from build123d import *

# Parameters (mm, degrees)
SKETCH1_R           = 10.5
BOSS_EXTRUDE1_DEPTH = 4.75
CUT_EXTRUDE1_DEPTH  = 5
CIRPATTERN1_COUNT   = 15


with BuildPart() as part:
    # Sketch1 → Boss-Extrude1 (new body)
    with BuildSketch(Plane(origin=(0, 0, 0), x_dir=(1, 0, 0), z_dir=(0, 1, 0))):
        with Locations(Location((0, 0, 0), (0, 0, 270))):
            Circle(SKETCH1_R)
        Polygon((4.734272207, 0), (2.367136104, 4.1), (-2.367136104, 4.1), (-4.734272207, 0), (-2.367136104, -4.1), (2.367136104, -4.1), align=None, mode=Mode.SUBTRACT)
    extrude(amount=BOSS_EXTRUDE1_DEPTH)

    # Sketch2 → Cut-Extrude1 (cut)
    with BuildSketch(Plane(origin=(0, 4.75, 0), x_dir=(1, 0, 0), z_dir=(0, 1, 0))):
        with BuildLine():
            Line((0, 5.75), (0, 9.700877125))
            Line((0, 9.700877125), (-0.75, 9.700877125))
            Line((-0.75, 9.700877125), (-0.75, 5.700877125))
            ThreePointArc((-0.75, 5.700877125), (-0.375803491, 5.737706139), (0, 5.75))
        make_face()
        with BuildLine():
            Line((0.75, 9.700877125), (0, 9.700877125))
            Line((0, 9.700877125), (0, 5.75))
            ThreePointArc((0, 5.75), (0.375803491, 5.737706139), (0.75, 5.700877125))
            Line((0.75, 5.700877125), (0.75, 9.700877125))
        make_face()
    cut_extrude1 = extrude(amount=-CUT_EXTRUDE1_DEPTH, mode=Mode.SUBTRACT)

    # CirPattern1: Cut-Extrude1 ×15 about axis
    cirpattern1_axis = Axis((0, 0, 0), (0, 1, 0))
    for i in range(1, CIRPATTERN1_COUNT):
        add(cut_extrude1.rotate(cirpattern1_axis, i * 360 / CIRPATTERN1_COUNT), mode=Mode.SUBTRACT)


solid = part.part
Check sheet for the modelled part. Datum: model origin and axes. Units: mm. Give positions to 0.01 mm unless a question says otherwise; leave off trailing zeros. Loops run counter-clockwise (first coordinate to the right, second up) from the corner with the lowest first, then second, coordinate; pieces in that order, holes last. Notation, with made-up numbers: M 40.5,87 L 89.5,87 A26 cw 89.5,113 Z; hole C 24,-11 d2. An arc over 180 degrees is marked long. Answer as a JSON object with one key per item and string values. Group by question number.
Q1. Material ranges on line 1 along X through (y, z) = (0.95, 4.5); line 2 along X through (y, z) = (1.2, -8); line 3 along Z through (x, y) = (7.75, 1.8), recorded low to high. Write a range as [from, to].
Q2. Cross-section at A-A on z = 3.75. Record the cut outline in (x, y).
Q3. Cross-section at B-B on y = 2.7. Give the number of separate pieces and of enclosed holes in the cut face, then the cut area to 3 significant figures.
Q4. Release check for a two-part mould opening along Z. For faces 1 (the flat face through (-3.936, 2.408, -8.866)), 2 (the flat face through (3.806, 2.408, -6.704)), 3 (the flat face through (0, 4.75, 5)) record: released by +Z, released by -Z, zero draft, split by the parting line, or undercut.
Q5. Go/stop test with flat-tipped pins: P1, Ø2, axis at x = -6.5, y = 4.5, coming from the -Z side; P2, Ø2, axis at y = 1, z = -2, coming from the -X side; P3, Ø2, axis at x = -3, y = 1.5, coming from the +Z side; P4, Ø4, axis at x = 2.5, z = -1.5, coming from the +Y side. Record where each tip stops, or that it passes through.
Evaluation:
{
 "1": {"line 1": "x = [-9.49, -8.6], [-6.29, -4.2], [-3.58, 3.58], [4.2, 6.29], [8.6, 9.49]", "line 2": "x = [-6.8, -4.38], [-2.74, -0.75], [0.75, 2.74], [4.38, 6.8]", "line 3": "z = [-7.08, -3.31], [-1.73, 0.06], [1.57, 3.61], [5.34, 7.08]"},
 "2": {"outline": "M -9.81,0 L -8,0 L -8,4.75 L -9.81,4.75 Z; M -5,0 L -2.57,0 L -2.57,4.75 L -5,4.75 Z; M 2.57,0 L 5,0 L 5,4.75 L 2.57,4.75 Z; M 8,0 L 9.81,0 L 9.81,4.75 L 8,4.75 Z"},
 "3": {"separate pieces": "1", "enclosed holes": "16", "area": "199 mm2"},
 "4": {"face 1": "undercut", "face 2": "undercut", "face 3": "zero draft"},
 "5": {"P1": "stops at z = -8.94", "P2": "stops at x = -10.45", "P3": "stops at z = 10.31", "P4": "stops at y = 4.75"}
}
